Geometry check sheet. Reference: the model listing, model coordinates, mm. Coordinates: 2 decimals unless noted, no trailing zeros. Write each loop counter-clockwise with the first axis right and the second up, starting at its lowest first coordinate (ties: lowest second). Pieces come first, ordered by that corner, then holes. Notation, with made-up numbers: (26.25, -11) -> (30.25, -11) arc R12 cw to (30.25, -6) -> close; hole circle Ø7 at (41, 88.5). An arc over 180 degrees is marked (long way). Answer in a Markdown table with one row per item. Add a question column.
1. Cross-section at D-D on y = 15.5. Record the cut outline in (x, z), and give its area (3 significant figures).
2. Depth check by flat-ended pin: P1, Ø1, axis at x = -2, y = 18.5, coming from the +Z side (3 decimals). Enter the tip coordinate at first touch or a pass-through.
3. Cross-section at C-C on x = 3.25. Record the cut outline in (y, z), and give its area (3 significant figures).
4. Mould release check, pull along Z, two halves, no side actions. Record for faces 1 (the cylindrical face through (0, 31, 0)), 2 (the cylindrical face through (0.07, 1.586, 18.214)), 3 (the flat face through (0, -11, 0)): pulls with the +Z half, pulls with the -Z half, needs draft (parallel to the pull), parting line crosses it, or undercut.
5. Scan lines: L1, parallel to Z at x = -3.5, y = 11; L2, parallel to Z at x = 2.5, y = 2.5; L3, parallel to Z at x = -1.25, y = 1.5. Record each from-to range of solid material in increasing order. Write a range as from..to.
6. Cross-section at B-B on y = 4.05. Record the cut outline in (x, z), and give its area (3 significant figures).
7. Cross-section at A-A on z = 0. Record the cut outline in (x, y).
Autodesk Inventor part; units mm, degrees
ref_plane "YZ Plane" through (0, 0, 0) normal (1, 0, 0) x (0, 1, 0)
ref_plane "XZ Plane" through (0, 0, 0) normal (0, 1, 0) x (-1, 0, 0)
ref_plane "XY Plane" through (0, 0, 0) normal (0, 0, 1) x (1, 0, 0)
sketch "Sketch1" plane through (0, 0, 0) normal (1, 0, 0) x (0, 1, 0)
  line L0 (-11, -20) -> (11, -20)
  arc A0 (11, -20) -> (11, 20) centre (11, 0) ccw
  line L1 (11, 20) -> (-11, 20)
  line L2 (-11, 20) -> (-11, -20)
  circle A1 centre (11, 0) radius 7.5
  point P0 (0, 0)
  point P1 (0, -20)
  dimension "d0" = 22
  dimension "d1" = 22
  dimension "d2" = 40
  dimension "d3" = 15
extrude "Extrusion1" add sketch "Sketch1" along normal mid plane 10
sketch "Sketch2" plane through (5, 0, 0) normal (1, 0, 0) x (0, 0, -1)
  arc A0 (20, 11) -> (-20, 11) centre (0, 11) ccw construction
  line L0 (-20, 11) -> (-20, -11) construction
  line L1 (-20, -11) -> (20, -11) construction
  line L2 (20, -11) -> (20, 11) construction
  circle A1 centre (0, 11) radius 7.5 construction
  circle A2 centre (15, 4.05) radius 4.05
  line L3 (0, 11) -> (0, -11) construction
  line L4 (-20, -11) -> (20, -11) construction
  circle A3 centre (-15, 4.05) radius 4.05
  point P0 (0, 0)
  dimension "d6" = 15.05
  dimension "d7" = 8.1
  dimension "d8" = 5
extrude "Extrusion2" cut sketch "Sketch2" against normal through all
properties part number "arco_obj4"
Results found:
| question | item | result |
|---|---|---|
| 1 | outline | (-5, -19.49) -> (5, -19.49) -> (5, -6) -> (-5, -6) -> close; (-5, 6) -> (5, 6) -> (5, 19.49) -> (-5, 19.49) -> close |
| 1 | area | 270 mm^2 |
| 2 | P1 | stops at z = 18.735 |
| 3 | outline | (-11, -20) -> (11, -20) arc R20 ccw to (11, 20) -> (-11, 20) -> close; hole circle Ø8.1 at (4.05, -15); hole circle Ø8.1 at (4.05, 15); hole circle Ø15 at (11, 0) |
| 3 | area | 1,230 mm^2 |
| 4 | face 1 | parting line crosses it |
| 4 | face 2 | undercut |
| 4 | face 3 | needs draft |
| 5 | L1 | z = -20..-7.5, 7.5..20 |
| 5 | L2 | z = -20..-18.74, -11.26..11.26, 18.74..20 |
| 5 | L3 | z = -20..-18.15, -11.85..11.85, 18.15..20 |
| 6 | outline | (-5, -20) -> (5, -20) -> (5, -19.05) -> (-5, -19.05) -> close; (-5, -10.95) -> (5, -10.95) -> (5, -2.82) -> (-5, -2.82) -> close; (-5, 2.82) -> (5, 2.82) -> (5, 10.95) -> (-5, 10.95) -> close; (-5, 19.05) -> (5, 19.05) -> (5, 20) -> (-5, 20) -> close |
| 6 | area | 182 mm^2 |
| 7 | outline | (-5, -11) -> (5, -11) -> (5, 3.5) -> (-5, 3.5) -> close; (-5, 18.5) -> (5, 18.5) -> (5, 31) -> (-5, 31) -> close |
